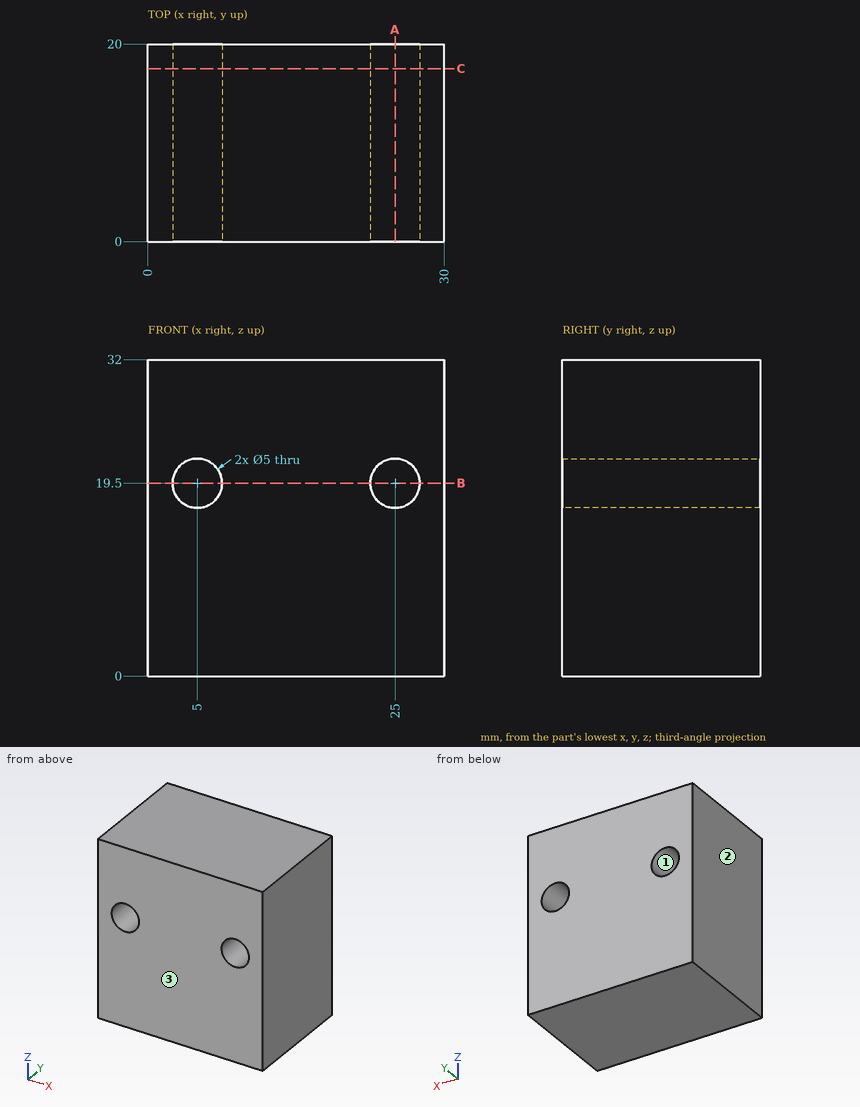
Drawing for the job (mm, zero at the part's lowest x, y, z). Round coordinates to 2 decimals unless told otherwise and drop trailing zeros. Order: outer loops, then holes, each group sorted by start corner. A loop starts at its lowest first (then second) coordinate and runs counter-clockwise, first axis right, second up.
Item 1: Probe line 1 along X through (y, z) = (8.5, 19.5); line 2 along X through (y, z) = (2.75, 21.5); line 3 along Z through (x, y) = (25, 10). List the from-to ranges inside material, lowest first.
Item 2: Saw through at B-B on z = 19.5. Write the cut outline in (x, y), then the cut area to 3 significant figures.
Item 3: Saw through at A-A on x = 25. Write the cut outline in (y, z).
Item 4: Saw through at C-C on y = 17.5. Write the cut outline in (x, z), then the cut area to 3 significant figures.
Item 5: Mould opens along X. For the marked faces 1, 2 and 3 say: pulls with the +X half, pulls with the -X half, needs draft (parallel to the pull), parting line crosses it, or undercut.
Reported:
1. line 1: x = 0 to 2.5, 7.5 to 22.5, 27.5 to 30
1. line 2: x = 0 to 3.5, 6.5 to 23.5, 26.5 to 30
1. line 3: z = 0 to 17, 22 to 32
2. outline: (0, 0) - (2.5, 0) - (2.5, 20) - (0, 20) - close; (7.5, 0) - (22.5, 0) - (22.5, 20) - (7.5, 20) - close; (27.5, 0) - (30, 0) - (30, 20) - (27.5, 20) - close
2. area: 400 mm2
3. outline: (0, 0) - (20, 0) - (20, 17) - (0, 17) - close; (0, 22) - (20, 22) - (20, 32) - (0, 32) - close
4. outline: (0, 0) - (30, 0) - (30, 32) - (0, 32) - close; hole circle Ø5 at (5, 19.5); hole circle Ø5 at (25, 19.5)
4. area: 921 mm2
5. face 1: undercut
5. face 2: pulls with the -X half
5. face 3: needs draft
